```python
from build123d import *

# Parameters (mm, degrees)
SKETCH_1_R               = 0.5
EXTRUDE_1_DEPTH          = 9.7
HOLE_WIZARD_M3_1_D       = 2.5
HOLE_WIZARD_M3_1_DEPTH   = 7.5
HOLE_WIZARD_M3_1_TIP     = 0.751075774
CUT_EXTRUDE_2_DEPTH      = 33.35053134
CHAMFER_1_SIZE           = 0.5
CHAMFER_2_SIZE           = 0.2
SKETCH_11_W              = 20
SKETCH_11_H              = 12
CUT_EXTRUDE_3_DEPTH      = 3.2
FILLET_2_R               = 1
FILLET_3_R               = 1
HOLE_WIZARD_M2_5_3_D     = 2.05
HOLE_WIZARD_M2_5_3_DEPTH = 8.35
HOLE_WIZARD_M2_5_3_TIP   = 0.615882135


with BuildPart() as part:
    # 草图1 → 凸台-拉伸1 (new body)
    with BuildSketch(Plane.XY):
        with BuildLine():
            Line((-22, 14.94880858), (22, 14.94880858))
            Line((22, 14.94880858), (24.5, 14.94880858))
            Line((24.5, 14.94880858), (27, -1.742947298))
            ThreePointArc((27, -1.742947298), (0, 0), (-27, -1.742947298))
            Line((-27, -1.742947298), (-24.5, 14.94880858))
            Line((-24.5, 14.94880858), (-22, 14.94880858))
        make_face()
        with Locations((-6, 6.94880858)):
            Circle(SKETCH_1_R, mode=Mode.SUBTRACT)
        with Locations((6, 6.94880858)):
            Circle(SKETCH_1_R, mode=Mode.SUBTRACT)
    extrude(amount=EXTRUDE_1_DEPTH)

    # M3 螺纹孔1
    with Locations(Plane(origin=(0, 14.94880858, 0), x_dir=(-1, 0, 0), z_dir=(0, 1, 0))):
        with Locations((-16.5, 3), (16.5, 3)):
            Hole(HOLE_WIZARD_M3_1_D / 2, depth=HOLE_WIZARD_M3_1_DEPTH)
            with Locations((0, 0, -(HOLE_WIZARD_M3_1_DEPTH + HOLE_WIZARD_M3_1_TIP / 2))):  # 118° drill point
                Cone(0, HOLE_WIZARD_M3_1_D / 2, HOLE_WIZARD_M3_1_TIP, mode=Mode.SUBTRACT)

    # 草图10 → 切除-拉伸2 (cut, through all)
    with BuildSketch(Plane.XY.offset(9.7)):
        Polygon((27, -1.742947298), (20.914837438, 15.00313582), (24.5, 14.94880858), align=None)
    cut_extrude_2 = extrude(amount=-CUT_EXTRUDE_2_DEPTH, mode=Mode.SUBTRACT)

    # 镜向1: 切除-拉伸2 across plane
    add(cut_extrude_2.mirror(Plane(origin=(0, 0, 0), x_dir=(0, 0, 1), z_dir=(1, 0, 0))), mode=Mode.SUBTRACT)

    # 倒角1
    chamfer_1_edges = [part.edges().sort_by_distance(p)[0] for p in [
        (-6.5, 6.94880858, 0),
        (-6.5, 6.94880858, 9.7),
        (5.5, 6.94880858, 0),
        (5.5, 6.94880858, 9.7),
    ]]
    chamfer(chamfer_1_edges, length=CHAMFER_1_SIZE)

    # 倒角2
    chamfer_2_edges = [part.edges().sort_by_distance(p)[0] for p in [
        (-17.75, 14.94880858, 3),
        (15.25, 14.94880858, 3),
    ]]
    chamfer(chamfer_2_edges, length=CHAMFER_2_SIZE)

    # 草图11 → 切除-拉伸3 (cut)
    with BuildSketch(Plane.XY.offset(9.7)):
        with Locations((0, 8.94880858)):
            Rectangle(SKETCH_11_W, SKETCH_11_H)
    extrude(amount=-CUT_EXTRUDE_3_DEPTH, mode=Mode.SUBTRACT)

    # 圆角2
    fillet_2_edges = [part.edges().sort_by_distance(p)[0] for p in [
        (-10, 8.94880858, 6.5),
        (-10, 2.94880858, 8.1),
        (0, 14.94880858, 6.5),
        (-10, 14.94880858, 8.1),
        (10, 8.94880858, 6.5),
        (10, 14.94880858, 8.1),
        (0, 2.94880858, 6.5),
        (10, 2.94880858, 8.1),
        (-10, 8.94880858, 9.7),
        (0, 2.94880858, 9.7),
        (10, 8.94880858, 9.7),
    ]]
    fillet(fillet_2_edges, radius=FILLET_2_R)

    # 圆角3
    fillet_3_edges = [part.edges().sort_by_distance(p)[0] for p in [
        (27, -1.742947298, 4.85),
        (-27, -1.742947298, 4.85),
        (0, 14.94880858, 0),
        (20.934578776, 14.94880858, 4.85),
        (23.967289388, 6.602930641, 0),
        (-20.934578776, 14.94880858, 4.85),
        (-23.967289388, 6.602930641, 0),
    ]]
    fillet(fillet_3_edges, radius=FILLET_3_R)

    # M2.5 螺纹孔3
    with Locations(Plane(origin=(6, 6.94880858, 6.5), x_dir=(1, 0, 0), z_dir=(0, 0, 1))):
        with Locations((0, 0), (-12, 0)):
            Hole(HOLE_WIZARD_M2_5_3_D / 2, depth=HOLE_WIZARD_M2_5_3_DEPTH)
            with Locations((0, 0, -(HOLE_WIZARD_M2_5_3_DEPTH + HOLE_WIZARD_M2_5_3_TIP / 2))):  # 118° drill point
                Cone(0, HOLE_WIZARD_M2_5_3_D / 2, HOLE_WIZARD_M2_5_3_TIP, mode=Mode.SUBTRACT)


solid = part.part
```
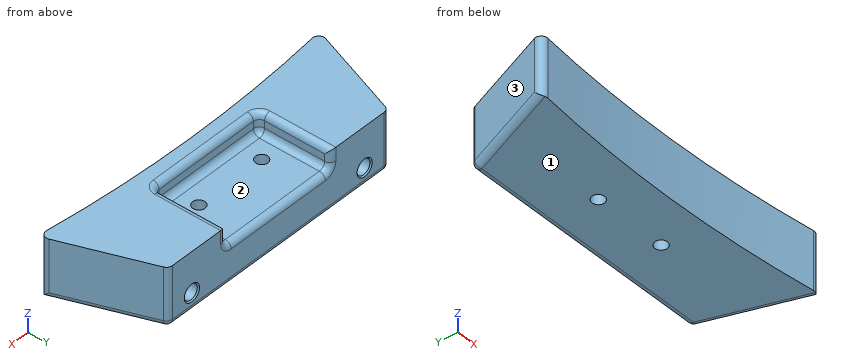
CAD build for the part. Positions are in the model's coordinates, mm. Face numbers are marked on the shaded views. Coordinates: 2 decimals unless noted, no trailing zeros. Write each loop counter-clockwise with the first axis right and the second up, starting at its lowest first coordinate (ties: lowest second). Pieces come first, ordered by that corner, then holes.
(1) Cut at C-C, the plane y = 11.25. Count the separate pieces of the cut face and the enclosed holes in it, and give its area (3 significant figures).
(2) Cut at B-B, the plane x = -6. List the corners of the cut face in (y, z).
(3) Cut at A-A, the plane z = 8. List the corners of the cut face in (x, y).
(4) Drill centre lines: probe 1 along Z at (x, y) = (16.5, 12.5); probe 2 along X at (y, z) = (12.25, 3); probe 3 along X at (y, z) = (7.25, 7.5). Where is each one in solid material? Low to high.
(5) Two-plate mould, pull along X, no slides. Class the marked faces 1, 2 and 3: +X half, -X half, draft (parallel to the pull), parting line (faces both ways), or undercut.
(6) Flat gauge pins, fed straight in: pin 1 (1 mm diameter, centred on y = 2, z = 8.5, fed in from -X); pin 2 (3 mm diameter, centred on x = -16.5, z = 3, fed in from +Y); pin 3 (1.3 mm diameter, centred on y = 11, z = 8, fed in from -X); pin 4 (1.5 mm diameter, centred on x = 16.5, z = 3, fed in from +Y). Where does each tip first touch, or does it go through?
Geometry says:
1. separate pieces: 1
1. enclosed holes: 2
1. area: 358 mm2
2. outline: (-0.09, 0) - (5.92, 0) - (5.92, 6.5) - (3.95, 6.5) arc R1 cw to (2.95, 7.5) - (2.95, 8.7) arc R1 ccw to (1.95, 9.7) - (-0.09, 9.7) - close; (7.97, 0) - (13.95, 0) arc R1 ccw to (14.95, 1) - (14.95, 5.5) arc R1 ccw to (13.95, 6.5) - (7.97, 6.5) - close
3. outline: (-26.44, -0.21) arc R1 ccw to (-25.38, -1.54) arc R210 cw to (25.38, -1.54) arc R1 ccw to (26.44, -0.21) - (21.17, 14.29) arc R1 ccw to (20.23, 14.95) - (11, 14.95) arc R1 ccw to (10, 13.95) - (10, 3.95) arc R1 cw to (9, 2.95) - (-9, 2.95) arc R1 cw to (-10, 3.95) - (-10, 13.95) arc R1 ccw to (-11, 14.95) - (-20.23, 14.95) arc R1 ccw to (-21.17, 14.29) - close
4. probe 1: z = 0 to 1.75, 4.25 to 9.7
4. probe 2: x = -21.92 to -17.75, -15.25 to 15.25, 17.75 to 21.92
4. probe 3: x = -23.73 to -10, 10 to 23.73
5. face 1: draft
5. face 2: undercut
5. face 3: -X half
6. pin 1: stops at x = -25.82
6. pin 2: stops at y = 14.95
6. pin 3: stops at x = -22.61
6. pin 4: stops at y = 7.15
